Verification items for the finished model (mm, model axes). Give positions to 0.01 mm unless a question says otherwise; leave off trailing zeros. Order: outer loops, then holes, each group sorted by start corner. A loop starts at its lowest first (then second) coordinate and runs counter-clockwise, first axis right, second up.
(1) Scan lines: L1, parallel to Z at x = -40, y = 4; L2, parallel to X at y = 5.25, z = -70; L3, parallel to Z at x = 75, y = 1.5. Record each from-to range of solid material in increasing order.
(2) Sectioned sample at B-B on z = 40. Record the cut outline in (x, y), plus the area to 3 significant figures.
(3) Sectioned sample at C-C on z = 0. Record the cut outline in (x, y).
(4) Sectioned sample at A-A on x = 0. Record the cut outline in (y, z), plus the area to 4 significant figures.
(5) Sectioned sample at D-D on x = -40. Record the cut outline in (y, z).
```python
from build123d import *

# Parameters (mm, degrees)
SKETCH2_W                                       = 170
SKETCH2_H                                       = 220
SKETCH2_R                                       = 35
SKETCH2_R_2                                     = 2.75
BOSS_EXTRUDE1_DEPTH                             = 6.35
CSK_FOR_M3_FLAT_HEAD_MACHINE_SCREW2_D           = 3.4
CSK_FOR_M3_FLAT_HEAD_MACHINE_SCREW2_CSINK_D     = 6.3
CSK_FOR_M3_FLAT_HEAD_MACHINE_SCREW2_CSINK_ANGLE = 90


with BuildPart() as part:
    # Sketch2 → Boss-Extrude1 (new body)
    with BuildSketch(Plane(origin=(0, 0, 0), x_dir=(1, 0, 0), z_dir=(0, 1, 0))):
        with Locations((0, -30)):
            Rectangle(SKETCH2_W, SKETCH2_H)
        Circle(SKETCH2_R, mode=Mode.SUBTRACT)
        with Locations((-40, 40)):
            Circle(SKETCH2_R_2, mode=Mode.SUBTRACT)
        with Locations((40, 40)):
            Circle(SKETCH2_R_2, mode=Mode.SUBTRACT)
        with Locations((40, -40)):
            Circle(SKETCH2_R_2, mode=Mode.SUBTRACT)
        with Locations((-40, -40)):
            Circle(SKETCH2_R_2, mode=Mode.SUBTRACT)
        with Locations((-75, 70)):
            Circle(SKETCH2_R_2, mode=Mode.SUBTRACT)
        with Locations((-75, -130)):
            Circle(SKETCH2_R_2, mode=Mode.SUBTRACT)
        with Locations((75, 70)):
            Circle(SKETCH2_R_2, mode=Mode.SUBTRACT)
        with Locations((75, -130)):
            Circle(SKETCH2_R_2, mode=Mode.SUBTRACT)
    extrude(amount=BOSS_EXTRUDE1_DEPTH)

    # CSK for M3 Flat Head Machine Screw2 (through all)
    with Locations(Plane(origin=(0, 0, 0), x_dir=(-1, 0, 0), z_dir=(0, -1, 0))):
        with Locations((57.523089764, -54.859977456), (-45.476910236, -54.859977456), (-32.976910236, -134.359977456), (49.523089764, -130.359977456)):
            CounterSinkHole(CSK_FOR_M3_FLAT_HEAD_MACHINE_SCREW2_D / 2, CSK_FOR_M3_FLAT_HEAD_MACHINE_SCREW2_CSINK_D / 2, counter_sink_angle=CSK_FOR_M3_FLAT_HEAD_MACHINE_SCREW2_CSINK_ANGLE)


solid = part.part
```
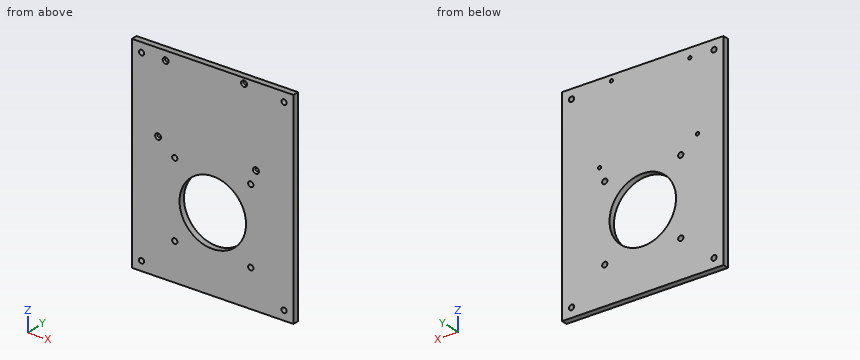
Ans:
1. L1: z = -80 to -42.75, -37.25 to 37.25, 42.75 to 140
1. L2: x = -85 to -77.75, -72.25 to 72.25, 77.75 to 85
1. L3: z = -80 to -72.75, -67.25 to 127.25, 132.75 to 140
2. outline: (-85, 0) - (-42.75, 0) - (-42.75, 6.35) - (-85, 6.35) - close; (-37.25, 0) - (37.25, 0) - (37.25, 6.35) - (-37.25, 6.35) - close; (42.75, 0) - (85, 0) - (85, 6.35) - (42.75, 6.35) - close
2. area: 1,010 mm2
3. outline: (-85, 0) - (-35, 0) - (-35, 6.35) - (-85, 6.35) - close; (35, 0) - (85, 0) - (85, 6.35) - (35, 6.35) - close
4. outline: (0, -80) - (6.35, -80) - (6.35, -35) - (0, -35) - close; (0, 35) - (6.35, 35) - (6.35, 140) - (0, 140) - close
4. area: 952.5 mm2
5. outline: (0, -80) - (6.35, -80) - (6.35, -42.75) - (0, -42.75) - close; (0, -37.25) - (6.35, -37.25) - (6.35, 37.25) - (0, 37.25) - close; (0, 42.75) - (6.35, 42.75) - (6.35, 140) - (0, 140) - close
